The listing builds one solid part. Answer for the finished solid, in the listing's coordinates (mm). A direction names the side the tool comes from. Round coordinates to 2 decimals unless told otherwise and drop trailing zeros. Write each loop counter-clockwise with the first axis right and the second up, starting at its lowest first coordinate (ties: lowest second). Pieces come first, ordered by that corner, then holes. Notation, with made-up numbers: M 74.5,60.25 L 90.5,60.25 A26 cw 90.5,92.25 Z; hole C -28,69 d7. An arc over 180 degrees is marked long. One line per item, written item: value. Start each with the question number.
(1) For faces 4 (the cylindrical face through (28.87, 12.97, 2.46)), 5 (the flat face through (7, 143, 2)), 6 (the flat face through (35, 147, 2)), determine the directions among +Z, -Z, +X, -X, +Y, -Y from which every point of the face is accessible in a straight line to the end or side of a thin tool.
(2) Consider probe 1 along Y at (x, z) = (22, 1.2); probe 2 along Y at (x, z) = (27, 2.65); probe 3 along X at (y, z) = (14, 3.5). Determine where each line is inside the solid, lowest interval first.
(3) Given P1, Ø4, axis at x = 10.39, y = 319.61, coming from the -Z side; P2, Ø1.5, axis at y = 149.5, z = 2, coming from the -X side; P3, Ø2.5, axis at y = 159, z = 3, coming from the +X side, each flat-ended and moving along its own axis, determine where each tip first touches the part or whether it passes through.
(4) Section B-B (z = 3.6) is taken. State how many separate pieces and enclosed holes the cut face has, plus the area to 3 significant figures.
(5) Section C-C (y = 116) is taken. Determine the outline of the cut face in (x, z).
(6) Section A-A (y = 14) is taken. Determine the outline of the cut face in (x, z).
(7) For a pull along X with two mould halves and no side action, classify faces 1 (the cylindrical face through (26.914, 318.275, 2.465)), 2 (the cylindrical face through (35.598, 292.784, 2.535)), 3 (the flat face through (21, 0, 3)) as released by +X, released by -X, zero draft, split by the parting line, or undercut.
```python
from build123d import *

# Parameters (mm, degrees)
SKETCH1_W              = 5
SKETCH1_H              = 330
BOSS_EXTRUDE1_DEPTH    = 42
CUT_EXTRUDE1_START     = -5
CUT_EXTRUDE1_OUTLINE_R = 11
CUT_EXTRUDE1_DEPTH     = 5
M4_CLEARANCE_HOLE1_D   = 4.5
CUT_EXTRUDE3_DEPTH     = 5
FILLET2_R              = 10
SKETCH10_R             = 7.9375
CUT_EXTRUDE4_DEPTH     = 5


# Read off the part's stored shape, not the designer's step: Cut-Extrude1
with BuildPart() as part:
    # Sketch1 → Boss-Extrude1 (new body)
    with BuildSketch(Plane(origin=(0, 0, 0), x_dir=(0, 0, -1), z_dir=(1, 0, 0))):
        with Locations((-2.5, 165)):
            Rectangle(SKETCH1_W, SKETCH1_H)
    extrude(amount=BOSS_EXTRUDE1_DEPTH)

    # Cut-Extrude1 outline → Cut-Extrude1 (cut)
    with BuildSketch(Plane.XY.offset(5).offset(CUT_EXTRUDE1_START)):
        with BuildLine():
            ThreePointArc((0, 309), (6.150757595, 323.849242405), (21, 330))
            Line((21, 330), (0, 330))
            Line((0, 330), (0, 309))
        make_face()
        with BuildLine():
            ThreePointArc((21, 330), (35.849242405, 323.849242405), (42, 309))
            Line((42, 309), (42, 330))
            Line((42, 330), (21, 330))
        make_face()
        with Locations((21, 309)):
            Circle(CUT_EXTRUDE1_OUTLINE_R)
    extrude(amount=CUT_EXTRUDE1_DEPTH, mode=Mode.SUBTRACT)

    # M4 Clearance Hole1 (through all)
    with Locations(Plane.XY.offset(5)):
        with Locations((10.393398282, 319.606601718), (31.606601718, 319.606601718), (31.606601718, 298.393398282), (10.393398282, 298.393398282)):
            Hole(M4_CLEARANCE_HOLE1_D / 2)

    # Sketch9 → Cut-Extrude3 (cut)
    with BuildSketch(Plane(origin=(0, 0, 0), x_dir=(-1, 0, 0), z_dir=(0, 0, -1))):
        with BuildLine():
            Line((-35, 293.347524158), (-35, 0))
            Line((-35, 0), (-42, 0))
            Line((-42, 0), (-42, 309))
            ThreePointArc((-42, 309), (-40.170289513, 300.4267859), (-35, 293.347524158))
        make_face()
        with BuildLine():
            Line((-7, 0), (-7, 293.347524158))
            ThreePointArc((-7, 293.347524158), (-1.829710487, 300.4267859), (0, 309))
            Line((0, 309), (0, 0))
            Line((0, 0), (-7, 0))
        make_face()
    extrude(amount=-CUT_EXTRUDE3_DEPTH, mode=Mode.SUBTRACT)

    # Fillet2
    fillet2_edges = [part.edges().sort_by_distance(p)[0] for p in [
        (35, 293.347524158, 2.5),
        (7, 293.347524158, 2.5),
    ]]
    fillet(fillet2_edges, radius=FILLET2_R)

    # Sketch10 → Cut-Extrude4 (cut)
    with BuildSketch(Plane(origin=(0, 0, 0), x_dir=(-1, 0, 0), z_dir=(0, 0, -1))):
        with Locations(Location((-21, 14, 0), (0, 0, 90))):
            Circle(SKETCH10_R)
    extrude(amount=-CUT_EXTRUDE4_DEPTH, mode=Mode.SUBTRACT)


solid = part.part
```
Recorded:
1. face 4: +Z, -Z
1. face 5: +Z, -Z, -X, -Y
1. face 6: +Z, -Z, +X, -Y
2. probe 1: y = 0 to 6.13, 21.87 to 298.05, 319.95 to 329.98
2. probe 2: y = 0 to 8.8, 19.2 to 299.78, 318.22 to 329.12
2. probe 3: x = 7 to 13.06, 28.94 to 35
3. P1: passes through
3. P2: stops at x = 7
3. P3: stops at x = 35
4. separate pieces: 1
4. enclosed holes: 6
4. area: 8,860 mm2
5. outline: M 7,0 L 35,0 L 35,5 L 7,5 Z
6. outline: M 7,0 L 13.06,0 L 13.06,5 L 7,5 Z; M 28.94,0 L 35,0 L 35,5 L 28.94,5 Z
7. face 1: undercut
7. face 2: released by +X
7. face 3: zero draft
